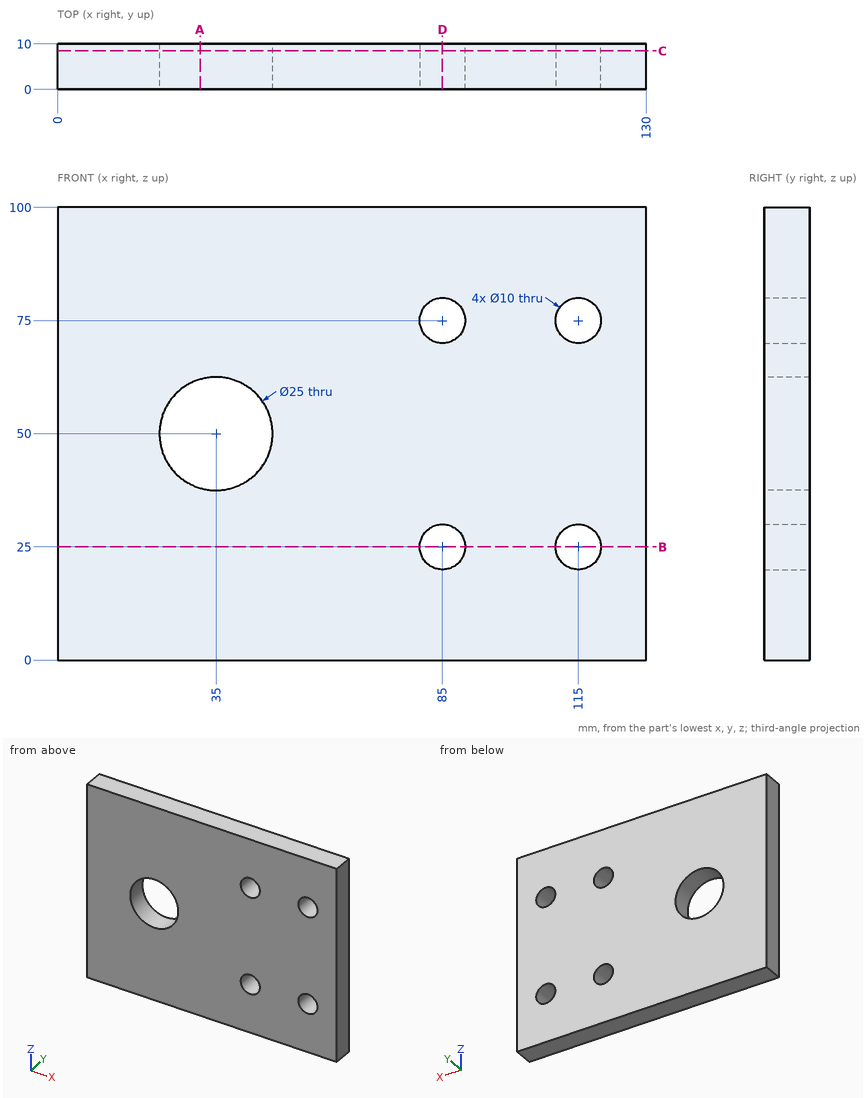
Could you check a few things on this drawing? It's one solid part, dimensions in mm from its lowest x, y, z. Round coordinates to 2 decimals unless told otherwise and drop trailing zeros. Loops run counter-clockwise (first coordinate to the right, second up) from the corner with the lowest first, then second, coordinate; pieces in that order, holes last. Notation, with made-up numbers: (66.25, 73.25) -> (106.25, 73.25) arc R28 ccw to (106.25, 95.25) -> close; hole circle Ø9 at (-26, 84.25). An arc over 180 degrees is marked (long way). One line per item, written item: value. Start each with the question number.
1. For pin 1 (9 mm diameter, centred on x = 115, z = 25, fed in from -Y), with a flat end and sliding along its axis, tell me the tip position at first contact or that it passes through.
2. If I drill on probe 1 along Z at (x, y) = (85, 7); probe 2 along Z at (x, y) = (35, 4); probe 3 along X at (y, z) = (8.5, 71), over which ranges is the centre line in solid material (lowest first)?
3. If we section it at C-C, the plane y = 8.5: Write out the boundary of the cut face in (x, z).
4. If we section it at A-A, the plane x = 31.5: Write out the boundary of the cut face in (y, z).
5. If we section it at D-D, the plane x = 85: Write out the boundary of the cut face in (y, z).
6. If we section it at B-B, the plane z = 25: Write out the boundary of the cut face in (x, y).
Calculated:
1. pin 1: passes through
2. probe 1: z = 0 to 20, 30 to 70, 80 to 100
2. probe 2: z = 0 to 37.5, 62.5 to 100
2. probe 3: x = 0 to 82, 88 to 112, 118 to 130
3. outline: (0, 0) -> (130, 0) -> (130, 100) -> (0, 100) -> close; hole circle Ø25 at (35, 50); hole circle Ø10 at (85, 25); hole circle Ø10 at (85, 75); hole circle Ø10 at (115, 25); hole circle Ø10 at (115, 75)
4. outline: (0, 0) -> (10, 0) -> (10, 38) -> (0, 38) -> close; (0, 62) -> (10, 62) -> (10, 100) -> (0, 100) -> close
5. outline: (0, 0) -> (10, 0) -> (10, 20) -> (0, 20) -> close; (0, 30) -> (10, 30) -> (10, 70) -> (0, 70) -> close; (0, 80) -> (10, 80) -> (10, 100) -> (0, 100) -> close
6. outline: (0, 0) -> (80, 0) -> (80, 10) -> (0, 10) -> close; (90, 0) -> (110, 0) -> (110, 10) -> (90, 10) -> close; (120, 0) -> (130, 0) -> (130, 10) -> (120, 10) -> close
